Model file for the job. Use its own axes, mm. Face numbers are marked on the shaded views. A direction names the side the tool comes from. Coordinates: 2 decimals unless noted, no trailing zeros. Write each loop counter-clockwise with the first axis right and the second up, starting at its lowest first coordinate (ties: lowest second). Pieces come first, ordered by that corner, then holes. Notation, with made-up numbers: M 67,46 L 86,46 A25 cw 86,75 Z; hole C -33,21 d2. An arc over 180 degrees is marked long. One line per question, with ' | ' between items. Start each with the question number.
(1) Two-plate mould, pull along Y, no slides. Class the marked faces 3, 4 and 5: +Y half, -Y half, draft (parallel to the pull), parting line (faces both ways), or undercut.
(2) Flat gauge pins, fed straight in: pin 1 Ø23 at (x, y) = (5.5, -20.5) entering from -Z; pin 2 Ø4 at (x, z) = (16, 11) entering from +Y; pin 3 Ø5 at (x, z) = (0.5, -17.5) entering from -Y. Where does each tip first touch, or does it go through?
(3) Wall check: probe 1 along X at (y, z) = (-45, -14.5); probe 2 along Y at (x, z) = (5, -4); probe 3 along Z at (x, y) = (19, -12). Give the ranges that are in metal, low to high.
(4) Cut at D-D (y = -22). Write the cut outline in (x, z), plus the area to 3 significant figures.
(5) Cut at C-C (z = 18.5). Write the cut outline in (x, y), plus the area to 3 significant figures.
(6) Cut at B-B (z = -17.5). Count the separate pieces of the cut face and the enclosed holes in it, plus the area to 3 significant figures.
(7) Tool access for the marked faces 1 and 2: list every direction of +Z, -Z, +X, -X, +Y, -Y with a clear straight run to the whole face (end or side of a thin tool).
(8) Cut at A-A (x = 9.5). Write the cut outline in (y, z).
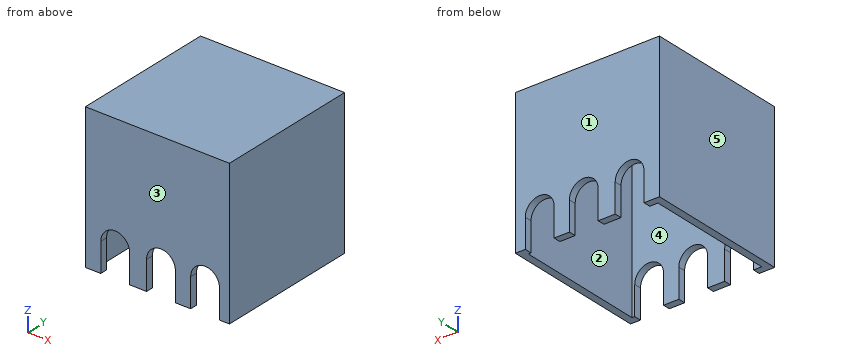
from build123d import *

# Parameters (mm, degrees)
F0_W     = 50.8
F0_H     = 50.8
F1_DEPTH = 50.8
F2_T     = -2.54
F3_W     = 10.16
F3_H     = 10.16
F4_DEPTH = 50.8


with BuildPart() as f1:
    # F0 (on Front) → F1 (new body)
    with BuildSketch(Plane.XZ):
        Rectangle(F0_W, F0_H)
    extrude(amount=F1_DEPTH)

    # F2
    f2_openings = [f1.faces().sort_by_distance(p)[0] for p in [
        (0, -25.4, -25.4),
    ]]
    offset(amount=F2_T, openings=f2_openings)

    # F3 (on face) → F4 (cut)
    with BuildSketch(Plane.XZ.offset(50.8)):
        with Locations((-14.884399, -20.32)):
            Rectangle(F3_W, F3_H)
        with BuildLine():
            ThreePointArc((-9.804399, -15.24), (-14.884399, -10.16), (-19.964399, -15.24))
            Line((-19.964399, -15.24), (-9.804399, -15.24))
        make_face()
        with Locations((1.270002, -20.32)):
            Rectangle(F3_W, F3_H)
        with BuildLine():
            ThreePointArc((6.350002, -15.24), (1.270002, -10.16), (-3.809998, -15.24))
            Line((-3.809998, -15.24), (6.350002, -15.24))
        make_face()
        with Locations((16.8148, -20.32)):
            Rectangle(F3_W, F3_H)
        with BuildLine():
            ThreePointArc((21.8948, -15.24), (16.8148, -10.16), (11.7348, -15.24))
            Line((11.7348, -15.24), (21.8948, -15.24))
        make_face()
    extrude(amount=-F4_DEPTH, mode=Mode.SUBTRACT)


solid = f1.part
Filled in:
1) face 3: -Y half | face 4: undercut | face 5: draft
2) pin 1: z = 22.86 | pin 2: y = 0 | pin 3: through
3) probe 1: -25.4 to -22.86, 22.86 to 25.4 | probe 2: -50.8 to -48.26, -2.54 to 0 | probe 3: 22.86 to 25.4
4) outline: M -25.4,-25.4 L -22.86,-25.4 L -22.86,22.86 L 22.86,22.86 L 22.86,-25.4 L 25.4,-25.4 L 25.4,25.4 L -25.4,25.4 Z | area: 374 mm²
5) outline: M -25.4,-50.8 L 25.4,-50.8 L 25.4,0 L -25.4,0 Z; hole M -22.86,-48.26 L 22.86,-48.26 L 22.86,-2.54 L -22.86,-2.54 Z | area: 490 mm²
6) separate pieces: 6 | enclosed holes: 0 | area: 335 mm²
7) face 1: +Z, -Z, +X, -X, +Y | face 2: -Z
8) outline: M -50.8,-25.4 L -48.26,-25.4 L -48.26,22.86 L -2.54,22.86 L -2.54,-25.4 L 0,-25.4 L 0,25.4 L -50.8,25.4 Z
